Autodesk Inventor part; units mm, degrees
ref_plane "YZ Plane" through (0, 0, 0) normal (1, 0, 0) x (0, 1, 0)
ref_plane "XZ Plane" through (0, 0, 0) normal (0, 1, 0) x (-1, 0, 0)
ref_plane "XY Plane" through (0, 0, 0) normal (0, 0, 1) x (1, 0, 0)
sketch "Sketch1" plane through (0, 0, 0) normal (0, 1, 0) x (-1, 0, 0)
  line L0 (0, 0) -> (44.45, 0)
  line L1 (44.45, 0) -> (44.45, 50.8)
  line L2 (44.45, 50.8) -> (0, 50.8)
  line L3 (0, 50.8) -> (0, 0)
  circle A0 centre (22.225, 25.4) radius 19.05
  line L4 (44.45, 25.4) -> (0, 25.4) construction
  line L5 (22.225, 50.8) -> (22.225, 0) construction
  line L6 (44.45, 0) -> (44.45, -3.175)
  line L7 (44.45, -3.175) -> (0, -3.175)
  line L8 (0, -3.175) -> (0, 0)
  arc A1 (44.45, 28.575) -> (22.225, 50.8) centre (22.225, 28.575) ccw
  arc A2 (22.225, -3.175) -> (44.45, 19.05) centre (22.225, 19.05) ccw
  line L9 (22.225, -3.175) -> (22.225, 0)
  dimension "d1" = 38.1
  dimension "d2" = 50.8
  dimension "d22" = 44.45
  dimension "d37" = 3.175
extrude "Extrusion1" add sketch "Sketch1" against normal blind 38.1 contours L3 L2 A1 L1 A2 L0 | L0 L9 L7 L8 | L0 A2 L9
sketch "Sketch3" plane through (0, 0, 0) normal (0, 1, 0) x (1, 0, 0)
  line L0 (-44.45, -19.05) -> (-44.45, -28.575)
  line L1 (-22.225, -50.8) -> (0, -50.8)
  line L2 (0, -50.8) -> (0, 3.175)
  circle A0 centre (-22.225, -25.4) radius 19.05
  circle A1 centre (-22.225, -25.4) radius 13.335
  circle A2 centre (-22.225, -9.906) radius 1.143
  circle A3 centre (-35.6432, -17.653) radius 1.143
  circle A4 centre (-35.6432, -33.147) radius 1.143
  circle A5 centre (-22.225, -40.894) radius 1.143
  circle A6 centre (-8.8068, -33.147) radius 1.143
  circle A7 centre (-8.8068, -17.653) radius 1.143
  line L3 (0, 3.175) -> (-22.225, 3.175)
  arc A8 (-22.225, 3.175) -> (-44.45, -19.05) centre (-22.225, -19.05) ccw
  arc A9 (-44.45, -28.575) -> (-22.225, -50.8) centre (-22.225, -28.575) ccw
  point P0 (0, 0)
  dimension "d6" = 26.67
  dimension "d7" = 2.286
  dimension "d8" = 15.494
  dimension "d11" = 360
extrude "Extrusion2" add sketch "Sketch3" along normal blind 3.175 contours A8 L3 L2 L1 A9 L0 | A0
sketch "Sketch4" plane through (0, 3.175, 0) normal (0, 1, 0) x (1, 0, 0)
  line L0 (-22.225, -50.8) -> (0, -50.8)
  line L1 (0, -50.8) -> (0, 3.175)
  line L2 (-44.45, -19.05) -> (-44.45, -28.575)
  circle A0 centre (-22.225, -25.4) radius 13.335
  circle A1 centre (-22.225, -9.906) radius 1.143
  circle A2 centre (-35.6432, -17.653) radius 1.143
  circle A3 centre (-35.6432, -33.147) radius 1.143
  circle A4 centre (-22.225, -40.894) radius 1.143
  circle A5 centre (-8.8068, -33.147) radius 1.143
  circle A6 centre (-8.8068, -17.653) radius 1.143
  line L3 (0, -25.4) -> (41.91, -25.4)
  line L4 (41.91, -25.4) -> (41.91, -50.8)
  line L5 (41.91, -50.8) -> (0, -50.8)
  line L6 (0, -50.8) -> (0, -25.4)
  circle A7 centre (10.16, -38.1) radius 2.286
  circle A8 centre (35.56, -38.1) radius 2.286
  line L7 (0, -38.1) -> (41.91, -38.1) construction
  arc A9 (29.21, -50.8) -> (29.21, -25.4) centre (29.21, -38.1) ccw
  arc A10 (0, -12.7) -> (12.7, -25.4) centre (12.7, -12.7) ccw
  arc A11 (-22.225, 3.175) -> (-44.45, -19.05) centre (-22.225, -19.05) ccw
  arc A12 (-44.45, -28.575) -> (-22.225, -50.8) centre (-22.225, -28.575) ccw
  line L8 (0, 3.175) -> (-22.225, 3.175)
  point P0 (0, 0)
  point P1 (0, -50.8)
  dimension "d15" = 10.16
  dimension "d16" = 25.4
  dimension "d17" = 4.572
  dimension "d18" = 25.4
  dimension "d19" = 6.35
  dimension "d30" = 12.7
extrude "Extrusion3" add sketch "Sketch4" against normal blind 3.175 contours L1 L3 A9 L5 | L1 A10 L3
sketch "Sketch6" plane through (0, -38.1, -3.175) normal (0, 0, -1) x (-1, 0, 0)
  line L0 (0, 0) -> (0, 41.275)
  line L1 (44.45, 0) -> (0, 0)
  line L2 (0, 41.275) -> (44.45, 41.275)
  line L3 (0, 19.05) -> (-17.78, 19.05)
  line L4 (-17.78, 19.05) -> (-17.78, 6.35)
  line L5 (-17.78, 6.35) -> (0, 6.35)
  line L6 (0, 6.35) -> (0, 19.05)
  circle A0 centre (-11.43, 12.7) radius 2.032
  line L7 (0, 12.7) -> (-17.78, 12.7) construction
  circle A1 centre (-11.43, 12.7) radius 6.35
  arc A2 (0, 0) -> (-11.43, 6.35) centre (-11.43, -7.112) ccw
  line L8 (0, 0) -> (0, 41.275)
  arc A3 (-11.43, 19.05) -> (0, 25.4) centre (-11.43, 32.512) ccw
  line L9 (44.45, 41.275) -> (44.45, 0)
  point P0 (0, 38.1)
  point P1 (0, 25.4)
  dimension "d24" = 11.43
  dimension "d25" = 4.064
  dimension "d26" = 6.35
  dimension "d27" = 6.35
  dimension "d36" = 25.4
extrude "Extrusion4" add sketch "Sketch6" against normal blind 3.175 contours A2 L5 L0 | L5 A1 L3 L0 | A1 | L3 A3 L0
fillet "Fillet2" [suppressed]
ref_plane "Work Plane1" through (0, -63.5, 0) normal (0, -1, 0) x (1, 0, 0)
mirror "Mirror1" about plane through (0, -63.5, 0) normal (0, -1, 0) of "Extrusion4", "Extrusion3", "Extrusion2", "Extrusion1"
sketch "Sketch7" plane through (0, -63.5, 0) normal (0, -1, 0) x (1, 0, 0)
  line L0 (-66.3836, -28.6153) -> (65.8055, -28.6153)
  line L1 (65.8055, -28.6153) -> (65.8055, 56.7488)
  line L2 (65.8055, 56.7488) -> (-66.3836, 56.7488)
  line L3 (-66.3836, 56.7488) -> (-66.3836, -28.6153)
  point P0 (0, 0)
extrude "Extrusion5" cut sketch "Sketch7" along normal through all
properties part number "Motor Mount right_3DPrint"
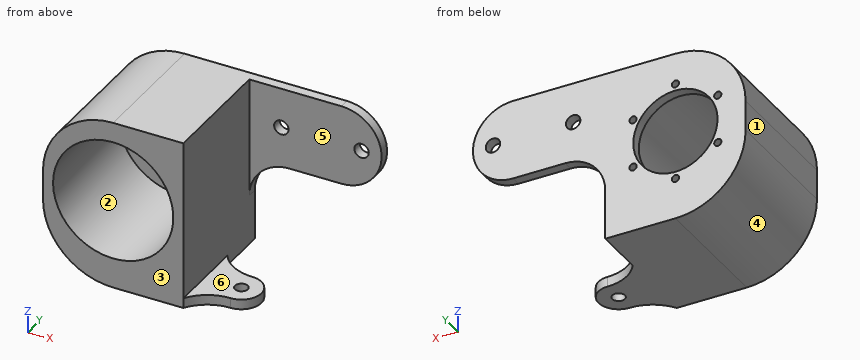
For this review, take the finished solid that the model builds, in its own axes (mm). Face numbers are marked on the shaded views. A direction names the side the tool comes from. Give positions to 0.01 mm unless a question says otherwise; leave off trailing zeros. Order: outer loops, then holes, each group sorted by start corner. A loop starts at its lowest first (then second) coordinate and runs counter-clockwise, first axis right, second up. Notation, with made-up numbers: (-1, 76.5) - (41, 76.5) arc R18 cw to (41, 80.5) - close; hole circle Ø8 at (-30.5, 35.25). An arc over 180 degrees is marked (long way). Answer as a JSON object with one key per item and string values. Group by question number.
Item 1: Wall thickness on line 1 along Y through (x, z) = (11.43, -1.9); line 2 along Z through (x, y) = (-22.5, -21); line 3 along X through (y, z) = (-28, 23.5): over which ranges is each line inside the solid? List them lowest first.
Item 2: Draft analysis for pull direction X (two halves, no side actions). For the marked faces 1, 2 and 3, state which applies: pulls with the +X half, pulls with the -X half, needs draft (parallel to the pull), parting line crosses it, or undercut.
Item 3: Clearance check with flat-ended pins moving along their axes: pin 1 Ø1 at (x, y) = (24.5, 1) entering from -Z; pin 2 Ø6 at (x, y) = (-35, -27) entering from -Z; pin 3 Ø2.5 at (x, z) = (-8.81, 17.65) entering from -Y. State where each tip first meets the part, or that it passes through.
Item 4: Take a section at D-D on z = 43. Give the boundary of the cut face in (x, y) (3 decimals), and give its area (3 significant figures).
Item 5: Take a section at A-A on y = -25.4. Give the boundary of the cut face in (x, z) (3 decimals), and give its area (3 significant figures).
Item 6: Machinability: for the marked faces 4, 5 and 6, which of the approach directions +Z, -Z, +X, -X, +Y, -Y give a long, thin tool a straight path to every point of the face, cutting with its end or side? Answer none if there is none.
Item 7: Take a section at C-C on x = -11. Give the boundary of the cut face in (y, z) (3 decimals).
Item 8: Take a section at B-B on y = -8.5. Give the boundary of the cut face in (x, z) (3 decimals), and give its area (3 significant figures).
Reported:
{
 "1": {"line 1": "-31.75 to -27.43, -23.37 to -19.05", "line 2": "-3.17 to 6.35, 44.45 to 50.8", "line 3": "-44.45 to -41.18, -3.27 to 0"},
 "2": {"face 1": "pulls with the -X half", "face 2": "undercut", "face 3": "needs draft"},
 "3": {"pin 1": "z = 25.4", "pin 2": "z = -0.91", "pin 3": "y = 0"},
 "4": {"outline": "(-39.133, -38.1) - (-29.515, -38.1) - (-29.515, 0) - (-14.935, 0) - (-14.935, -38.1) - (0, -38.1) - (0, 0) - (40.927, 0) - (40.927, 3.175) - (-39.133, 3.175) - close", "area": "1,190 mm^2"},
 "5": {"outline": "(-44.45, 19.05) arc R22.225 ccw to (-22.225, -3.175) - (9.398, -3.175) - (9.398, 0) - (0, 0) - (0, 50.8) - (-22.225, 50.8) arc R22.225 ccw to (-44.45, 28.575) - close; (13.462, -3.175) - (17.78, -3.175) - (17.78, 0) - (13.462, 0) - close; hole circle Ø38.1 at (-22.225, 25.4)", "area": "1,090 mm^2"},
 "6": {"face 4": "-Z, -X, +Y, -Y", "face 5": "+Z, -Z, +X, -Y", "face 6": "+Z, +X, +Y, -Y"},
 "7": {"outline": "(-38.1, -3.175) - (3.175, -3.175) - (3.175, 18.201) - (0, 18.201) - (0, 10.008) - (-38.1, 10.008) - close; (-38.1, 40.792) - (0, 40.792) - (0, 32.599) - (3.175, 32.599) - (3.175, 50.8) - (-38.1, 50.8) - close"},
 "8": {"outline": "(-44.45, 19.05) arc R22.225 ccw to (-22.225, -3.175) - (0, -3.175) - (0, 50.8) - (-22.225, 50.8) arc R22.225 ccw to (-44.45, 28.575) - close; hole circle Ø38.1 at (-22.225, 25.4)", "area": "1,050 mm^2"}
}
